Design review of the part built by this model. Coordinates are the model's own, in mm. Round coordinates to 2 decimals unless told otherwise and drop trailing zeros. Order: outer loops, then holes, each group sorted by start corner. A loop starts at its lowest first (then second) coordinate and runs counter-clockwise, first axis right, second up. Notation, with made-up numbers: M -31.75,54.5 L 25.25,54.5 A28 ccw 25.25,87.5 Z; hole C 30.5,52 d7. An arc over 180 degrees is marked long. Use a Markdown table: item, result. Add a question column.
(1) To check wall thickness, follow probe 1 along Z at (x, y) = (-34.5, 3.65); probe 2 along X at (y, z) = (1.9, -8.25); probe 3 along X at (y, z) = (4.15, -15.25). State the ranges of each line that lie inside material, in increasing order. Write a range as from..to.
(2) Take a section at B-B (y = 3.1). Count the separate pieces of the cut face and the enclosed holes in it, then the cut area to 3 significant figures.
(3) Take a section at A-A (z = 2). Write out the cut boundary in (x, y), then the cut area to 3 significant figures.
```python
from build123d import *

# Parameters (mm, degrees)
ESBO_O1_W                = 113
ESBO_O1_H                = 25
RESSALTO_EXTRUS_O1_DEPTH = 5
CORTE_EXTRUS_O1_DEPTH    = 5
ESBO_O4_R                = 1
ESBO_O4_R_2              = 1.1
CORTE_EXTRUS_O2_DEPTH    = 76
ESBO_O5_R                = 2
CORTE_EXTRUS_O3_DEPTH    = 10


with BuildPart() as part:
    # Esboço1 → Ressalto-extrusão1 (new body)
    with BuildSketch(Plane(origin=(0, 0, 0), x_dir=(1, 0, 0), z_dir=(0, 1, 0))):
        with Locations((9.231716451, 5.983979594)):
            Rectangle(ESBO_O1_W, ESBO_O1_H)
    extrude(amount=RESSALTO_EXTRUS_O1_DEPTH)

    # Esboço2 → Corte-extrusão1 (cut)
    with BuildSketch(Plane(origin=(0, 5, 0), x_dir=(1, 0, 0), z_dir=(0, 1, 0))):
        Polygon((65.731716451, 4.983979594), (62.231716451, 4.983979594), (62.231716451, 3.183979594), (60.731716451, 3.183979594), (60.731716451, 4.983979594), (58.731716451, 4.983979594), (58.731716451, 6.983979594), (60.731716451, 6.983979594), (60.731716451, 8.783979594), (62.231716451, 8.783979594), (62.231716451, 6.983979594), (65.731716451, 6.983979594), align=None)
    corte_extrus_o1 = extrude(amount=-CORTE_EXTRUS_O1_DEPTH, mode=Mode.SUBTRACT)

    # Espelhar1: Corte-extrusão1 across plane
    add(corte_extrus_o1.mirror(Plane(origin=(9.231716451, 0, 0), x_dir=(0, 0, 1), z_dir=(1, 0, 0))), mode=Mode.SUBTRACT)

    # Esboço4 → Corte-extrusão2 (cut)
    with BuildSketch(Plane(origin=(0, 5, 0), x_dir=(1, 0, 0), z_dir=(0, 1, 0))):
        with Locations(Location((-25.688283549, 12.683979594, 0), (0, 0, 270))):
            Circle(ESBO_O4_R)
        with Locations(Location((44.151716451, 12.683979594, 0), (0, 0, 270))):
            Circle(ESBO_O4_R_2)
    extrude(amount=-CORTE_EXTRUS_O2_DEPTH, mode=Mode.SUBTRACT)

    # Esboço5 → Corte-extrusão3 (cut)
    with BuildSketch(Plane(origin=(0, 5, 0), x_dir=(1, 0, 0), z_dir=(0, 1, 0))):
        with Locations(Location((-34.268283549, 13.483979594, 0), (0, 0, 270))):
            Circle(ESBO_O5_R)
        with Locations(Location((-34.268283549, -1.516020406, 0), (0, 0, 270))):
            Circle(ESBO_O5_R)
        with Locations(Location((52.731716451, 13.483979594, 0), (0, 0, 270))):
            Circle(ESBO_O5_R)
        with Locations(Location((52.731716451, -1.516020406, 0), (0, 0, 270))):
            Circle(ESBO_O5_R)
    extrude(amount=-CORTE_EXTRUS_O3_DEPTH, mode=Mode.SUBTRACT)


solid = part.part
```
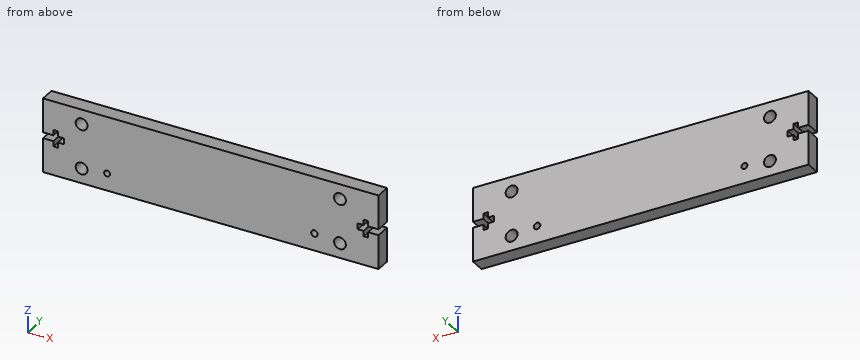
Verdict:
| question | item | result |
|---|---|---|
| 1 | probe 1 | z = -18.48..-15.47, -11.5..-0.47, 3.5..6.52 |
| 1 | probe 2 | x = -47.27..-43.77, -42.27..60.73, 62.23..65.73 |
| 1 | probe 3 | x = -47.27..-35.21, -33.33..51.79, 53.67..65.73 |
| 2 | separate pieces | 1 |
| 2 | enclosed holes | 6 |
| 2 | area | 2,730 mm^2 |
| 3 | outline | M -47.27,0 L -36.21,0 L -36.21,5 L -47.27,5 Z; M -32.33,0 L 50.79,0 L 50.79,5 L -32.33,5 Z; M 54.67,0 L 65.73,0 L 65.73,5 L 54.67,5 Z |
| 3 | area | 526 mm^2 |
